Input: part model. Units: mm. Frame: model coordinates. A direction names the side the tool comes from. Give positions to 0.01 mm unless a question says otherwise; leave off trailing zeros. Write each loop counter-clockwise with the first axis right and the second up, starting at its lowest first coordinate (ties: lowest second). Pieces come first, ordered by that corner, then holes.
```python
from build123d import *

# Parameters (mm, degrees)
PAD004_DEPTH = 4
SKETCH005_R  = 2
PAD005_DEPTH = 5
PAD006_DEPTH = 3
FILLET003_R  = 0.9
FILLET004_R  = 0.9


with BuildPart() as part:
    # Sketch004 → Pad004 (new body)
    with BuildSketch(Plane.XY):
        with BuildLine():
            ThreePointArc((3, -6), (0, -3), (-3, -6))
            Line((-3, -6), (-3, -16))
            ThreePointArc((-3, -16), (0, -19), (3, -16))
            Line((3, -6), (3, -16))
        make_face()
    extrude(amount=-PAD004_DEPTH)

    # Sketch005 → Pad005 (new body)
    with BuildSketch(Plane.XY):
        with Locations((0, -6)):
            Circle(SKETCH005_R)
    extrude(amount=PAD005_DEPTH)

    # Sketch006 → Pad006 (new body)
    with BuildSketch(Plane.XY.offset(5)):
        with BuildLine():
            ThreePointArc((3, -6), (0, -3), (-3, -6))
            Line((-3, -6), (-3, -12))
            ThreePointArc((-3, -12), (0, -15), (3, -12))
            Line((3, -6), (3, -12))
        make_face()
    extrude(amount=PAD006_DEPTH)

    # Fillet003
    fillet003_edges = [part.edges().sort_by_distance(p)[0] for p in [
        (-2, -6, 5),
    ]]
    fillet(fillet003_edges, radius=FILLET003_R)

    # Fillet004
    fillet004_edges = [part.edges().sort_by_distance(p)[0] for p in [
        (-2, -6, 0),
    ]]
    fillet(fillet004_edges, radius=FILLET004_R)


solid = part.part
```
Q1. Material intervals for line 1 along Z through (x, y) = (-0.95, -10.5); line 2 along Z through (x, y) = (0.9, -8.25); line 3 along Z through (x, y) = (-2.25, -14.25), sorted ascending.
Q2. Section D-D, the plane y = -14.5. Return the cut outline in (x, z), then the cut area to 3 significant figures.
Q3. Access query for faces 1 (the cylindrical face through (0, -19, -2)), 2 (the cylindrical face through (0, -8, 2)), 3 (the cylindrical face through (0, -15, 6)). Directions: +Z, -Z, +X, -X, +Y, -Y. A direction counts if a zero-diameter tool reaches every point of the face in a straight line with its end or side. Return the directions, or none.
Q4. Section B-B, the plane x = 0. Return the cut outline in (y, z).
Q5. Section A-A, the plane y = -9.75. Return the cut outline in (x, z), then the cut area to 3 significant figures.
Q6. Section C-C, the plane z = 3.25. Return the cut outline in (x, y).
Q7. Mould query, pull axis Z, two halves, no side actions, for faces 4 (the flat face through (0, -13, 0)), 5 (the flat face through (0, -9, 8)), 6 (the flat face through (0, -12, 5)), 7 (the flat face through (3, -9, 6)). Classes: +Z half, -Z half, draft (parallel to the pull), parting line (faces both ways), or undercut.
Q8. Pin query (flat end, axial travel): pin 1 (2 mm diameter, centred on x = -1, z = 1.5, fed in from -Y). Return the tip coordinate at first contact, or that it passes through.
Solutions:
1. line 1: z = -4 to 0, 5 to 8
1. line 2: z = -4 to 0.14, 4.86 to 8
1. line 3: z = -4 to 0
2. outline: (-3, -4) - (3, -4) - (3, 0) - (-3, 0) - close; (-1.66, 5) - (1.66, 5) - (1.66, 8) - (-1.66, 8) - close
2. area: 33.9 mm2
3. face 1: +Z, -Z, -Y
3. face 2: none
3. face 3: +Z, -Y
4. outline: (-19, -4) - (-3, -4) - (-3, 0) - (-3.1, 0) arc R0.9 cw to (-4, 0.9) - (-4, 4.1) arc R0.9 cw to (-3.1, 5) - (-3, 5) - (-3, 8) - (-15, 8) - (-15, 5) - (-8.9, 5) arc R0.9 cw to (-8, 4.1) - (-8, 0.9) arc R0.9 cw to (-8.9, 0) - (-19, 0) - close
5. outline: (-3, -4) - (3, -4) - (3, 0) - (-3, 0) - close; (-3, 5) - (3, 5) - (3, 8) - (-3, 8) - close
5. area: 42.0 mm2
6. outline: circle Ø4 at (0, -6)
7. face 4: undercut
7. face 5: +Z half
7. face 6: undercut
7. face 7: draft
8. pin 1: stops at y = -8
